from build123d import *

# Parameters (mm, degrees)
SKETCH2_W           = 6.35
SKETCH2_H           = 120.65
BOSS_EXTRUDE1_DEPTH = 3.81
EDGE_1_R            = 3.048
EDGE_2_R            = 3.048
EDGE_3_R            = 3.048
EDGE_4_R            = 3.048
SKETCH4_R           = 1.905
HOLES_DEPTH         = 121.877049517


with BuildPart() as part:
    # Sketch2 → Boss-Extrude1 (new body)
    with BuildSketch(Plane.XY):
        with Locations((3.175, 60.325)):
            Rectangle(SKETCH2_W, SKETCH2_H)
    extrude(amount=BOSS_EXTRUDE1_DEPTH)

    # Edge 1
    edge_1_edges = [part.edges().sort_by_distance(p)[0] for p in [
        (6.35, 120.65, 1.905),
    ]]
    fillet(edge_1_edges, radius=EDGE_1_R)

    # Edge 2
    edge_2_edges = [part.edges().sort_by_distance(p)[0] for p in [
        (0, 120.65, 1.905),
    ]]
    fillet(edge_2_edges, radius=EDGE_2_R)

    # Edge 3
    edge_3_edges = [part.edges().sort_by_distance(p)[0] for p in [
        (6.35, 0, 1.905),
    ]]
    fillet(edge_3_edges, radius=EDGE_3_R)

    # Edge 4
    edge_4_edges = [part.edges().sort_by_distance(p)[0] for p in [
        (0, 0, 1.905),
    ]]
    fillet(edge_4_edges, radius=EDGE_4_R)

    # Sketch4 → Holes (cut, through all)
    with BuildSketch(Plane.XY.offset(3.81)):
        with Locations((3.175, 3.175)):
            Circle(SKETCH4_R)
        with Locations((3.175, 117.475)):
            Circle(SKETCH4_R)
    extrude(amount=-HOLES_DEPTH, mode=Mode.SUBTRACT)


solid = part.part
Design review of the part built by this model. Coordinates are the model's own, in mm. Round coordinates to 2 decimals unless told otherwise and drop trailing zeros. Write each loop counter-clockwise with the first axis right and the second up, starting at its lowest first coordinate (ties: lowest second). Pieces come first, ordered by that corner, then holes.
Item 1: Consider section A-A on z = 1.25. Give the boundary of the cut face in (x, y) (3 decimals), and give its area (3 significant figures).
Item 2: Wall thickness on L1, parallel to Y at x = 3, z = 0.8; L2, parallel to Y at x = 4.25, z = 1.75; L3, parallel to Y at x = 1, z = 2.75: over which ranges is each line inside the solid? List them lowest first.
Item 3: Draft analysis for pull direction X (two halves, no side actions). For faces 1 (the cylindrical face through (2.927, 5.064, 1.932)), 2 (the cylindrical face through (5.481, 119.733, 1.932)), 3 (the flat face through (0, 60, 2)), state which applies: released by +X, released by -X, zero draft, split by the parting line, or undercut.
Item 4: For pin 1 Ø3 at (x, y) = (2, 13) entering from -Z, flat-tipped, find the tip position at first contact; note if it passes through.
Check values:
1. outline: (0, 3.048) arc R3.048 ccw to (3.048, 0) - (3.302, 0) arc R3.048 ccw to (6.35, 3.048) - (6.35, 117.602) arc R3.048 ccw to (3.302, 120.65) - (3.048, 120.65) arc R3.048 ccw to (0, 117.602) - close; hole circle Ø3.81 at (3.175, 3.175); hole circle Ø3.81 at (3.175, 117.475)
1. area: 735 mm2
2. L1: y = 0 to 1.28, 5.07 to 115.58, 119.37 to 120.65
2. L2: y = 0.15 to 1.6, 4.75 to 115.9, 119.05 to 120.5
2. L3: y = 0.79 to 119.86
3. face 1: undercut
3. face 2: released by +X
3. face 3: released by -X
4. pin 1: stops at z = 0
